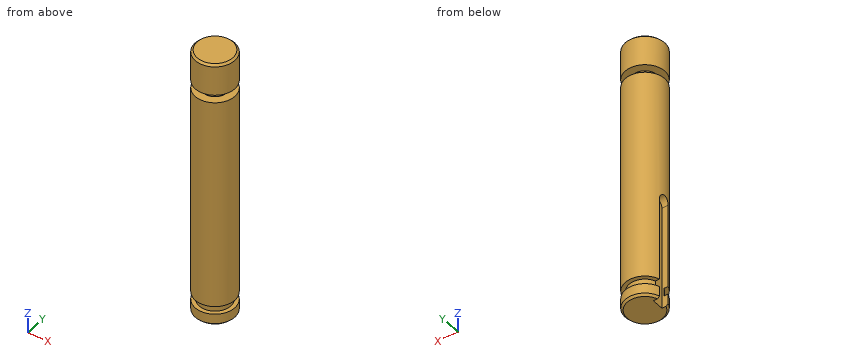
```python
from build123d import *

# Parameters (mm, degrees)
SKETCH1_R           = 5
BOSS_EXTRUDE1_DEPTH = 34.5
CUT_EXTRUDE1_START  = -10
SKETCH2_R           = 5
SKETCH2_R_2         = 3
CUT_EXTRUDE1_DEPTH  = 2
CUT_EXTRUDE2_START  = -5
SKETCH4_R           = 5
SKETCH4_R_2         = 4
CUT_EXTRUDE2_DEPTH  = 2
CHAMFER1_SIZE       = 0.5
CUT_EXTRUDE4_START  = -3.2
CUT_EXTRUDE4_DEPTH  = 2.8


with BuildPart() as part:
    # Sketch1 → Boss-Extrude1 (new body, symmetric)
    with BuildSketch(Plane.XY):
        Circle(SKETCH1_R)
    extrude(amount=BOSS_EXTRUDE1_DEPTH, both=True)

    # Sketch2 → Cut-Extrude1 (cut)
    with BuildSketch(Plane.XY.offset(34.5).offset(CUT_EXTRUDE1_START)):
        Circle(SKETCH2_R)
        Circle(SKETCH2_R_2, mode=Mode.SUBTRACT)
    extrude(amount=CUT_EXTRUDE1_DEPTH, mode=Mode.SUBTRACT)

    # Sketch4 → Cut-Extrude2 (cut)
    with BuildSketch(Plane(origin=(0, 0, -34.5), x_dir=(-1, 0, 0), z_dir=(0, 0, -1)).offset(CUT_EXTRUDE2_START)):
        Circle(SKETCH4_R)
        Circle(SKETCH4_R_2, mode=Mode.SUBTRACT)
    extrude(amount=CUT_EXTRUDE2_DEPTH, mode=Mode.SUBTRACT)

    # Chamfer1
    chamfer1_edges = [part.edges().sort_by_distance(p)[0] for p in [
        (-5, 0, -34.5),
        (-5, 0, 34.5),
    ]]
    chamfer(chamfer1_edges, length=CHAMFER1_SIZE)

    # Sketch7 → Cut-Extrude4 (cut, through all)
    with BuildSketch(Plane(origin=(0, 0, 0), x_dir=(0, 0, -1), z_dir=(1, 0, 0)).offset(CUT_EXTRUDE4_START)):
        with BuildLine():
            Line((8, 1.5), (34.5, 1.5))
            Line((34.5, 1.5), (34.5, -1.5))
            Line((34.5, -1.5), (8, -1.5))
            ThreePointArc((8, -1.5), (6.5, 0), (8, 1.5))
        make_face()
    extrude(amount=-CUT_EXTRUDE4_DEPTH, mode=Mode.SUBTRACT)


solid = part.part
```
Input: part model. Units: mm. Frame: model coordinates. Round coordinates to 2 decimals unless told otherwise and drop trailing zeros. Loops run counter-clockwise (first coordinate to the right, second up) from the corner with the lowest first, then second, coordinate; pieces in that order, holes last.
1) Section query C-C on z = -11.5. Return the cut outline in (x, y).
Ans:
outline: (-4.77, -1.5) arc R5 ccw (long way) to (-4.77, 1.5) - (-3.2, 1.5) - (-3.2, -1.5) - close
2) Section query A-A on y = 0. Return the cut outline in (x, z).
Ans:
outline: (-5, -6.5) - (-3.2, -6.5) - (-3.2, -34.5) - (4.5, -34.5) - (5, -34) - (5, -31.5) - (4, -31.5) - (4, -29.5) - (5, -29.5) - (5, 24.5) - (3, 24.5) - (3, 26.5) - (5, 26.5) - (5, 34) - (4.5, 34.5) - (-4.5, 34.5) - (-5, 34) - (-5, 26.5) - (-3, 26.5) - (-3, 24.5) - (-5, 24.5) - close
3) Section query D-D on z = 13.5. Return the cut outline in (x, y).
Ans:
outline: circle Ø10 at (0, 0)
4) Material intervals for line 1 (Z direction, x = 3.5, y = -0.25); line 2 (Z direction, x = 3.75, y = -2.75); line 3 (X direction, y = 3, z = -13.5), sorted ascending.
Ans:
line 1: z = -34.5 to 24.5, 26.5 to 34.5
line 2: z = -34.35 to -31.5, -29.5 to 24.5, 26.5 to 34.35
line 3: x = -4 to 4
5) Section query B-B on x = 0. Return the cut outline in (y, z), plus the area to 4 significant figures.
Ans:
outline: (-5, -34) - (-4.5, -34.5) - (4.5, -34.5) - (5, -34) - (5, -31.5) - (4, -31.5) - (4, -29.5) - (5, -29.5) - (5, 24.5) - (3, 24.5) - (3, 26.5) - (5, 26.5) - (5, 34) - (4.5, 34.5) - (-4.5, 34.5) - (-5, 34) - (-5, 26.5) - (-3, 26.5) - (-3, 24.5) - (-5, 24.5) - (-5, -29.5) - (-4, -29.5) - (-4, -31.5) - (-5, -31.5) - close
area: 677.5 mm2
6) Pin query (flat end, axial travel): pin 1 (1.3 mm diameter, centred on x = -3.5, z = -23.5, fed in from +Y); pin 2 (0.5 mm diameter, centred on x = -4, z = -19.5, fed in from -Y); pin 3 (2 mm diameter, centred on x = -1.5, z = 18.5, fed in from -Y). Return the tip coordinate at first contact, or that it passes through.
Ans:
pin 1: stops at y = 4.11
pin 2: stops at y = -3.31
pin 3: stops at y = -4.97
